Autodesk Inventor part; units mm, degrees
ref_plane "YZ Plane" through (0, 0, 0) normal (1, 0, 0) x (0, 1, 0)
ref_plane "XZ Plane" through (0, 0, 0) normal (0, 1, 0) x (-1, 0, 0)
ref_plane "XY Plane" through (0, 0, 0) normal (0, 0, 1) x (1, 0, 0)
sketch "Skizze1" plane through (0, 0, 0) normal (0, 0, 1) x (1, 0, 0)
  circle A0 centre (0, 0) radius 6.5
  line L0 (-27, 12) -> (27, 12)
  line L1 (27, 12) -> (27, -12)
  line L2 (27, -12) -> (-27, -12)
  line L3 (-27, -12) -> (-27, 12)
  dimension "d0" = 13
  dimension "d1" = 24
  dimension "d2" = 12
  dimension "d3" = 54
  dimension "d4" = 27
extrude "Extrusion1" add sketch "Skizze1" along normal blind 4
sketch "Skizze2" plane through (0, 0, 0) normal (0, 0, -1) x (-1, 0, 0)
  line L0 (-27, -12) -> (-13, -12)
  line L1 (-13, -12) -> (-13, 12)
  line L2 (-13, 12) -> (-27, 12)
  line L3 (-27, 12) -> (-27, -12)
  line L4 (13, -12) -> (27, -12)
  line L5 (27, -12) -> (27, 12)
  line L6 (27, 12) -> (13, 12)
  line L7 (13, 12) -> (13, -12)
  point P0 (0, 0)
  dimension "d7" = 14
  dimension "d8" = 14
  dimension "d9" = 24
  dimension "d10" = 24
  dimension "d11" = 27
  dimension "d12" = 27
  dimension "d13" = 12
extrude "Extrusion2" add sketch "Skizze2" along normal blind 14
hole "Bohrung1" at (20, 12, -7) direction (0, -1, 0) diameter 6.1 depth 24
hole "Bohrung2" at (-20, 12, -7) direction (0, -1, 0) diameter 6.1 depth 724
hole "Bohrung3" at (-9, 0, 4) direction (0, 0, -1) diameter 3 depth 8 tip angle 118
pattern_circular "Runde Anordnung1" count 3 over 360 about axis through (0, 0, 0) along (0, 0, 1) of "Bohrung3"
properties part number "B Arm"
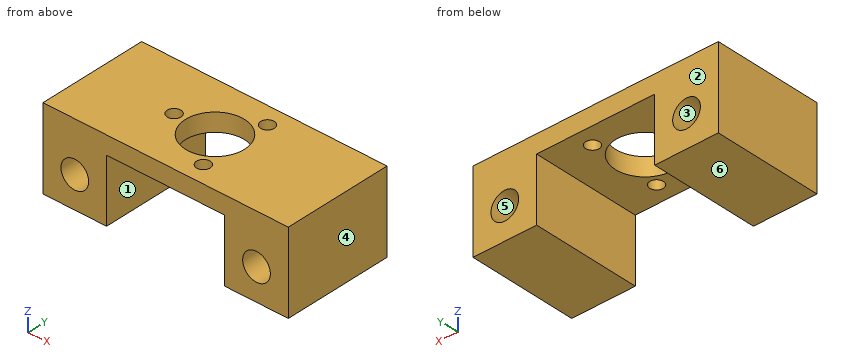
Geometry check sheet. Reference: the model listing, model coordinates, mm. Face numbers are marked on the shaded views. A direction names the side the tool comes from. Give positions to 0.01 mm unless a question says otherwise; leave off trailing zeros. Loops run counter-clockwise (first coordinate to the right, second up) from the corner with the lowest first, then second, coordinate; pieces in that order, holes last. Notation, with made-up numbers: M 8.25,89 L 64.25,89 A16 cw 64.25,94 Z; hole C 26.5,-13 d3. An arc over 180 degrees is marked long. Write item = value, one per line. Start each with the question number.
1. Section check D-D, the plane z = -0.5. Enter the section's corners in (x, y), plus the area to 3 significant figures.
2. Draft check along Z on the marked faces 3, 4, 5 and 6. Enter one of: +Z half, -Z half, draft (parallel to the pull), parting line (faces both ways), or undercut.
3. Go/stop test with flat-tipped pins: P1, Ø10.5, axis at x = 0, y = 0, coming from the +Z side; P2, Ø4, axis at x = -9, y = 0, coming from the -Z side. Record where each tip stops, or that it passes through.
4. Section check B-B, the plane z = -7. Enter the section's corners in (x, y), plus the area to 3 significant figures.
5. Thickness scan on probe 1 along X at (y, z) = (-4.5, -7); probe 2 along Z at (x, y) = (20, -4.5); probe 3 along X at (y, z) = (-7.25, -11.5). Record the ranges inside material, lowest first.
6. Section check C-C, the plane y = 0. Enter the section's corners in (x, z), plus the area to 3 significant figures.
7. Tool access check on the marked faces 1 and 2. Record the directions out of +Z, -Z, +X, -X, +Y, -Y that give a thin tool (end or side, any length) a straight path to the whole face; none if there is none.
8. Section check A-A, the plane x = 0. Enter the section's corners in (y, z), plus the area to 3 significant figures.
Values follow:
q1.outline = M -27,-12 L -13,-12 L -13,12 L -27,12 Z; M 13,-12 L 27,-12 L 27,12 L 13,12 Z
q1.area = 672 mm^2
q2.face_3 = undercut
q2.face_4 = draft
q2.face_5 = undercut
q2.face_6 = -Z half
q3.P1 = through
q3.P2 = 0
q4.outline = M -27,-12 L -23.05,-12 L -23.05,12 L -27,12 Z; M -16.95,-12 L -13,-12 L -13,12 L -16.95,12 Z; M 13,-12 L 16.95,-12 L 16.95,12 L 13,12 Z; M 23.05,-12 L 27,-12 L 27,12 L 23.05,12 Z
q4.area = 379 mm^2
q5.probe_1 = -27 to -23.05, -16.95 to -13, 13 to 16.95, 23.05 to 27
q5.probe_2 = -14 to -10.05, -3.95 to 4
q5.probe_3 = -27 to -13, 13 to 27
q6.outline = M -27,-14 L -13,-14 L -13,0 L -10.5,0 L -10.5,4 L -27,4 Z; M -7.5,0 L -6.5,0 L -6.5,4 L -7.5,4 Z; M 6.5,0 L 13,0 L 13,-14 L 27,-14 L 27,4 L 6.5,4 Z; hole C -20,-7 d6.1; hole C 20,-7 d6.1
q6.area = 486 mm^2
q7.face_1 = -Z, +Y, -Y
q7.face_2 = +Z, -Z, +X, -X, +Y
q8.outline = M -12,0 L -6.5,0 L -6.5,4 L -12,4 Z; M 6.5,0 L 12,0 L 12,4 L 6.5,4 Z
q8.area = 44.0 mm^2
